Geometry check sheet. Reference: the model listing, model coordinates, mm. Give positions to 0.01 mm unless a question says otherwise; leave off trailing zeros. Loops run counter-clockwise (first coordinate to the right, second up) from the corner with the lowest first, then second, coordinate; pieces in that order, holes last.
```python
from build123d import *

# Parameters (mm, degrees)
BOSS_EXTRUDE1_DEPTH = 450.85
SKETCH2_W           = 22.225
SKETCH2_H           = 3.175
CUT_EXTRUDE1_DEPTH  = 26.4


with BuildPart() as part:
    # Sketch1 → Boss-Extrude1 (new body)
    with BuildSketch(Plane.XY):
        Polygon((0, 0), (0, 25.4), (3.175, 25.4), (3.175, 3.175), (25.4, 3.175), (25.4, 0), align=None)
    extrude(amount=BOSS_EXTRUDE1_DEPTH)

    # Sketch2 → Cut-Extrude1 (cut, through all)
    with BuildSketch(Plane(origin=(25.4, 0, 0), x_dir=(0, 0, -1), z_dir=(1, 0, 0))):
        with Locations((-439.7375, 1.5875)):
            Rectangle(SKETCH2_W, SKETCH2_H)
        with Locations((-11.1125, 1.5875)):
            Rectangle(SKETCH2_W, SKETCH2_H)
    extrude(amount=-CUT_EXTRUDE1_DEPTH, mode=Mode.SUBTRACT)


solid = part.part
```
1) Sectioned sample at B-B on x = 16. Enter the section's corners in (y, z) (3 decimals), plus the area to 3 significant figures.
2) Depth check by flat-ended pin: P1, Ø6, axis at y = 17, z = 184.5, coming from the +X side (3 decimals); P2, Ø2, axis at x = 5, z = 399.5, coming from the +Y side (3 decimals); P3, Ø3.5, axis at x = 1, z = 15.5, coming from the -Y side (3 decimals). Enter the tip coordinate at first touch or a pass-through.
3) Sectioned sample at C-C on y = 17.25. Enter the section's corners in (x, z) (3 decimals).
4) Sectioned sample at A-A on z = 90.5. Enter the section's corners in (x, y) (3 decimals), plus the area to 3 significant figures.
5) Scan lines: line 1 along X through (y, z) = (15, 431) (3 decimals); line 2 along Z through (x, y) = (19.75, 1.5) (3 decimals). Record each from-to range of solid material in increasing order.
6) Mould release check, pull along Y, two halves, no side actions. Record for faces 1 (the flat face through (13, 0, 223)), 2 (the flat face through (0, 13, 222)), 3 (the flat face through (14, 3.175, 223)): +Y half, -Y half, draft (parallel to the pull), parting line (faces both ways), or undercut.
Determined:
1. outline: (0, 22.225) - (3.175, 22.225) - (3.175, 428.625) - (0, 428.625) - close
1. area: 1,290 mm2
2. P1: stops at x = 3.175
2. P2: stops at y = 3.175
2. P3: stops at y = 3.175
3. outline: (0, 0) - (3.175, 0) - (3.175, 450.85) - (0, 450.85) - close
4. outline: (0, 0) - (25.4, 0) - (25.4, 3.175) - (3.175, 3.175) - (3.175, 25.4) - (0, 25.4) - close
4. area: 151 mm2
5. line 1: x = 0 to 3.175
5. line 2: z = 22.225 to 428.625
6. face 1: -Y half
6. face 2: draft
6. face 3: +Y half
